Could you check a few things on this model? Use its own coordinates, in mm. Round coordinates to 2 decimals unless told otherwise and drop trailing zeros. Loops run counter-clockwise (first coordinate to the right, second up) from the corner with the lowest first, then second, coordinate; pieces in that order, holes last. Notation, with made-up numbers: (22, 22) -> (27, 22) arc R13 cw to (27, 39) -> close; hole circle Ø10 at (5, -27.5). An arc over 180 degrees is marked (long way). Use CSV: the item, a comma, the result in double quotes. Start each with the question number.
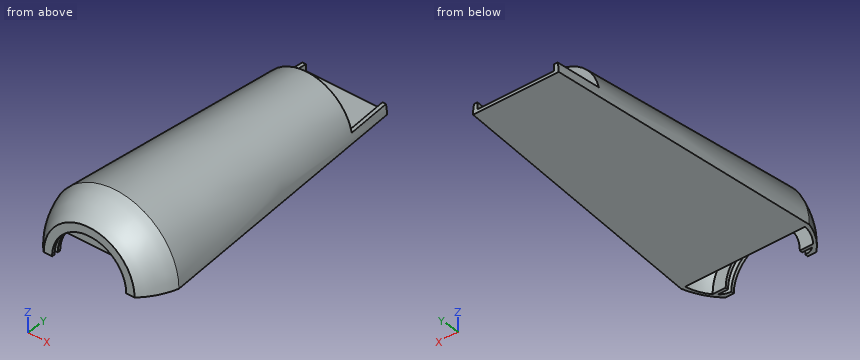
```python
from build123d import *

# Parameters (mm, degrees)
REVOLVE1_ANGLE = 180


with BuildPart() as part:
    # Sketch1 → Revolve1 (revolve)
    with BuildSketch(Plane.XY):
        with BuildLine():
            Line((27.686, 0), (22.606, 0))
            Line((22.606, 0), (22.606, 1.8288))
            add(Edge.make_bspline(
                [(22.606, 1.8288), (25.041168082, 1.8288), (27.106875675, 2.820982452), (28.829, 4.191)],
                knots=[0, 0, 0, 0, 0.286842678, 0.286842678, 0.286842678, 0.286842678], degree=3))
            Line((28.829, 4.191), (22.606, 4.191))
            Line((22.606, 4.191), (22.606, 5.8928))
            Line((22.606, 5.8928), (30.607, 5.8928))
            add(Edge.make_bspline(
                [(30.607, 5.8928), (35.326430108, 11.240557446), (36.542913871, 18.669)],
                knots=[0.392904056, 0.392904056, 0.392904056, 1, 1, 1], degree=2))
            Line((36.542913871, 18.669), (0, 18.669))
            Line((0, 18.669), (0, 185.547))
            Line((0, 185.547), (26.0985, 185.547))
            Line((26.0985, 185.547), (39.0906, 18.669))
            add(Edge.make_bspline(
                [(27.686, 0), (33.019237831, 4.973324735), (36.732929961, 10.734198825), (39.0906, 18.669)],
                knots=[0, 0, 0, 0, 1, 1, 1, 1], degree=3))
        make_face()
    revolve(axis=Axis((0, 18.669, 0), (0, -1, 0)), revolution_arc=REVOLVE1_ANGLE)

    # Sketch2 for Cut-Loft1 → Cut-Loft1 section 0
    with BuildSketch(Plane(origin=(0, 185.547, 0), x_dir=(1, 0, 0), z_dir=(0, 1, 0))):
        with BuildLine():
            Line((-23.3045, -1.778), (23.3045, -1.778))
            Line((23.3045, -1.778), (23.3045, -5.842))
            Line((23.3045, -5.842), (25.43624851, -5.842))
            Line((25.43624851, -5.842), (28.03631071, -5.842))
            # circular arc as an exact rational Bezier (weights 1, cos(half-angle), 1)
            Bezier((28.03631071, -5.842), (0, -140.390907609), (-28.03631071, -5.842), weights=[1, 0.203991131, 1])
            Line((-28.03631071, -5.842), (-25.43624851, -5.842))
            Line((-25.43624851, -5.842), (-23.3045, -5.842))
            Line((-23.3045, -5.842), (-23.3045, -1.778))
        make_face()
    # Sketch4 for Cut-Loft1 → Cut-Loft1 section 1
    with BuildSketch(Plane(origin=(0, 158.115, 0), x_dir=(1, 0, 0), z_dir=(0, 1, 0))):
        with BuildLine():
            Line((-25.491437213, -1.778), (25.491437213, -1.778))
            Line((25.491437213, -1.778), (25.491437213, -5.842))
            Line((25.491437213, -5.842), (27.623185722, -5.842))
            Line((27.623185722, -5.842), (30.214593541, -5.842))
            Bezier((30.214593541, -5.842), (0, -162.110685865), (-30.214593541, -5.842), weights=[1, 0.189834418, 1])
            Line((-30.214593541, -5.842), (-27.623185722, -5.842))
            Line((-27.623185722, -5.842), (-25.491437213, -5.842))
            Line((-25.491437213, -5.842), (-25.491437213, -1.778))
        make_face()
    loft(mode=Mode.SUBTRACT)


solid = part.part
```
1. Suppose I cut it at A-A (y = 145.5). List the corners of the cut face in (x, z) for me.
2. If I drill on L1, parallel to Y at x = -21, z = 13 (3 decimals); L2, parallel to Y at x = -1, z = 5 (3 decimals); L3, parallel to X at y = 164.5, z = 3.5, over which ranges is the centre line in solid material (lowest first)?
3. Will these pins go through, and if not, where does the flat tip stop? pin 1 (12 mm diameter, centred on y = 141.5, z = 20.5, fed in from -X); pin 2 (14.5 mm diameter, centred on x = 13.5, z = 19.5, fed in from -Y); pin 3 (6 mm diameter, centred on y = 39, z = 7, fed in from -X); pin 4 (4 mm diameter, centred on x = -11, y = 163.5, fed in from +Z).
4. Suppose I cut it at B-B (y = 109). List the corners of the cut face in (x, z) for me, then the cut area to 3 significant figures.
Geometry check:
1,outline,"(-29.22, 0) -> (29.22, 0) arc R29.22 ccw to start"
2,L1,"y = 0 to 2.08, 4.191 to 5.893, 18.669 to 158.115"
2,L2,"y = 18.669 to 158.115"
2,L3,"x = -27.52 to -24.98, 24.98 to 27.52"
3,pin 1,"stops at x = -25.76"
3,pin 2,"stops at y = 0"
3,pin 3,"stops at x = -37.37"
3,pin 4,"stops at z = 1.78"
4,outline,"(-32.06, 0) -> (32.06, 0) arc R32.06 ccw to start"
4,area,"1,610 mm²"
